from build123d import *

# Parameters (mm, degrees)
BOX002_W            = 8
BOX002_H            = 2
BOX002_DEPTH        = 0.2
BOX001_W            = 8
BOX001_H            = 2
BOX001_DEPTH        = 0.2
BOX_W               = 30
BOX_H               = 17
BOX_DEPTH           = 4.5
BOX_PLACEMENT_ANGLE = 90
FILLET_R            = 1


with BuildPart() as box002:
    # Box002 → Box002 (new body)
    with BuildSketch(Plane(origin=(49.15, -57, 0), x_dir=(0, 0, 1), z_dir=(0, -1, 0))):
        with Locations((4, 1)):
            Rectangle(BOX002_W, BOX002_H)
    extrude(amount=BOX002_DEPTH)


with BuildPart() as box001:
    # Box001 → Box001 (new body)
    with BuildSketch(Plane(origin=(42.65, -57, 0), x_dir=(0, 0, 1), z_dir=(0, -1, 0))):
        with Locations((4, 1)):
            Rectangle(BOX001_W, BOX001_H)
    extrude(amount=BOX001_DEPTH)


with BuildPart() as battery:
    # Box → Box (new body)
    with BuildSketch(Plane.XY):
        with Locations((15, 8.5)):
            Rectangle(BOX_W, BOX_H)
    extrude(amount=BOX_DEPTH)


with BuildPart() as battery_1:
    # Box placement: moved
    add(battery.part.moved(Location((53.5, -57, 4.75))).rotate(Axis((53.5, -57, 4.75), (0, 0, 1)), BOX_PLACEMENT_ANGLE))

    # Fillet
    fillet_edges = [battery_1.edges().sort_by_distance(p)[0] for p in [
        (53.5, -57, 7),
        (45, -57, 9.25),
        (36.5, -57, 7),
        (45, -57, 4.75),
        (53.5, -27, 7),
        (45, -27, 9.25),
        (36.5, -27, 7),
        (45, -27, 4.75),
        (53.5, -42, 4.75),
        (53.5, -42, 9.25),
        (36.5, -42, 4.75),
        (36.5, -42, 9.25),
    ]]
    fillet(fillet_edges, radius=FILLET_R)

    # Fusion: union Box002, Box001
    add(box002.part)
    add(box001.part)


solid = battery_1.part
The model under review builds one solid part; all positions refer to its coordinate system, in mm. A direction names the side the tool comes from. Coordinates: 2 decimals unless noted, no trailing zeros. Loops run counter-clockwise (first coordinate to the right, second up) from the corner with the lowest first, then second, coordinate; pieces in that order, holes last. Notation, with made-up numbers: M -6.75,-6 L 20.25,-6 A19 cw 20.25,6 Z; hole C 2.25,80.25 d4. An arc over 180 degrees is marked long. Put each result on its own line as item: value. Start each with the question number.
Q1. Add section C-C (y = -53). Write out the cut boundary in (x, z), and give its area (3 significant figures).
Q2. Wall thickness on line 1 (Y direction, x = 41.75, z = 4); line 2 (Y direction, x = 50.25, z = 7.75); line 3 (Z direction, x = 46.25, y = -31): over which ranges is each line inside the solid? List them lowest first.
Q3. For faces 1 (the cylindrical face through (36.801, -27.285, 7.018)), 2 (the flat face through (45, -42, 4.75)), list the 3-axis set-ups (+Z, -Z, +X, -X, +Y, -Y) from which the entire face can be reached by the end or side of a thin tool; tool diameter is ignored.
Q4. Clearance check with flat-ended pins moving along their axes: pin 1 (5 mm diameter, centred on y = -36, z = 5.5, fed in from +X); pin 2 (1 mm diameter, centred on x = 42, z = 4, fed in from +Y); pin 3 (2 mm diameter, centred on x = 48.5, z = 4, fed in from +Y); pin 4 (1 mm diameter, centred on x = 42.5, y = -50.5, fed in from -Z). State where each tip first meets the part, or that it passes through.
Q5. Add section A-A (z = 2.5). Write out the cut boundary in (x, y).
Q6. Add section B-B (x = 43). Write out the cut boundary in (y, z).
Q7. The part is to be moulded in two halves that separate along Y. For faces 3 (the flat face through (42, -57, 3)), 4 (the cylindrical face through (53.199, -56.715, 7.018)), 5 (the flat face through (45, -42, 9.25)), say which applies: +Y half, -Y half, draft (parallel to the pull), parting line (faces both ways), or undercut.
Answers:
1. outline: M 36.5,5.75 A1 ccw 37.5,4.75 L 52.5,4.75 A1 ccw 53.5,5.75 L 53.5,8.25 A1 ccw 52.5,9.25 L 37.5,9.25 A1 ccw 36.5,8.25 Z
1. area: 75.6 mm^2
2. line 1: y = -57.2 to -57
2. line 2: y = -57 to -27
2. line 3: z = 4.75 to 9.25
3. face 1: +Z, -Z, -X, +Y
3. face 2: -Z, +X, -X, +Y
4. pin 1: stops at x = 53.5
4. pin 2: stops at y = -57
4. pin 3: stops at y = -27.34
4. pin 4: stops at z = 4.75
5. outline: M 40.65,-57.2 L 42.65,-57.2 L 42.65,-57 L 40.65,-57 Z; M 47.15,-57.2 L 49.15,-57.2 L 49.15,-57 L 47.15,-57 Z
6. outline: M -57,5.75 A1 ccw -56,4.75 L -28,4.75 A1 ccw -27,5.75 L -27,8.25 A1 ccw -28,9.25 L -56,9.25 A1 ccw -57,8.25 Z
7. face 3: undercut
7. face 4: -Y half
7. face 5: draft
